Check sheet for the modelled part. Datum: model origin and axes. Units: mm. A direction names the side the tool comes from. Coordinates: 2 decimals unless noted, no trailing zeros. Write each loop counter-clockwise with the first axis right and the second up, starting at its lowest first coordinate (ties: lowest second). Pieces come first, ordered by that corner, then holes. Notation, with made-up numbers: (25.25, 12.5) - (44.25, 12.5) arc R24 ccw to (44.25, 51.5) - close; hole circle Ø9 at (-26.5, -31.75). An arc over 180 degrees is marked (long way). Use one line per item in the form item = value. Start each with the question number.
1. Tool access check on faces 4 (the face through (14, 15.57, 0.99)), 5 (the face through (7.5, 5, 4)), 6 (the face through (-7.5, 5, 4)), 7 (the face through (-9, 21, 10)). Record the directions out of +Z, -Z, +X, -X, +Y, -Y that give a thin tool (end or side, any length) a straight path to the whole face; none if there is none.
2. Cross-section at C-C on x = 0. Record the boundary of the cut face in (y, z).
3. Cross-section at D-D on z = 3.25. Record the boundary of the cut face in (x, y).
4. Cross-section at A-A on z = 16. Record the boundary of the cut face in (x, y).
5. Scan lines: line 1 along Y through (x, z) = (-15.5, 1.55); line 2 along Y through (x, z) = (-3.5, 4.5); line 3 along Y through (x, z) = (-17, 10.5). Record each from-to range of solid material in increasing order.
6. Draft check along Y on faces 1 (the face through (-21, 0, 19)), 2 (the face through (0, 2, 2)), 3 (the face through (0, -23, 10)). Enter one of: +Y half, -Y half, draft (parallel to the pull), parting line (faces both ways), or undercut.
7. Cross-section at B-B on y = 0. Record the boundary of the cut face in (x, z).
8. Go/stop test with flat-tipped pins: pin 1 Ø2.5 at (x, y) = (15.5, 15.5) entering from -Z; pin 2 Ø2 at (y, z) = (5.5, 4) entering from -X; pin 3 Ø1 at (x, z) = (-3, 4) entering from +Y. Record where each tip stops, or that it passes through.
```python
from build123d import *

# Parameters (mm, degrees)
F0_W     = 42
F0_H     = 46
F0_R     = 1.5
F1_DEPTH = 2
F2_W     = 12
F2_H     = 3
F2_W_2   = 42
F3_DEPTH = 16
F4_W     = 42
F4_H     = 46
F4_R     = 2
F4_R_2   = 18
F5_DEPTH = 2
F6_W     = 15
F6_H     = 2
F7_DEPTH = 4
F8_SIZE  = 0.5


with BuildPart() as f1:
    # F0 (on Top) → F1 (new body)
    with BuildSketch(Plane.XY):
        Rectangle(F0_W, F0_H)
        with Locations((-15.5, -15.5)):
            Circle(F0_R, mode=Mode.SUBTRACT)
        with Locations((15.5, -15.5)):
            Circle(F0_R, mode=Mode.SUBTRACT)
        with Locations((-15.5, 15.5)):
            Circle(F0_R, mode=Mode.SUBTRACT)
        with Locations((15.5, 15.5)):
            Circle(F0_R, mode=Mode.SUBTRACT)
    extrude(amount=F1_DEPTH)

    # F2 (on face) → F3 (join)
    with BuildSketch(Plane.XY.offset(2)):
        with Locations((15, 21.5)):
            Rectangle(F2_W, F2_H)
        with Locations((-15, 21.5)):
            Rectangle(F2_W, F2_H)
        with Locations((0, -21.5)):
            Rectangle(F2_W_2, F2_H)
    extrude(amount=F3_DEPTH)

    # F4 (on face) → F5 (join)
    with BuildSketch(Plane.XY.offset(18)):
        Rectangle(F4_W, F4_H)
        with Locations((-16, -18)):
            Circle(F4_R, mode=Mode.SUBTRACT)
        with Locations((16, -18)):
            Circle(F4_R, mode=Mode.SUBTRACT)
        with Locations((-16, 18)):
            Circle(F4_R, mode=Mode.SUBTRACT)
        Circle(F4_R_2, mode=Mode.SUBTRACT)
        with Locations((16, 18)):
            Circle(F4_R, mode=Mode.SUBTRACT)
    extrude(amount=F5_DEPTH)

    # F6 (on face) → F7 (join)
    with BuildSketch(Plane.XY.offset(2)):
        with Locations((0, 9)):
            Rectangle(F6_W, F6_H)
        with Locations((0, 5.5)):
            Rectangle(F6_W, F6_H)
    extrude(amount=F7_DEPTH)

    # F8
    f8_edges = [f1.edges().sort_by_distance(p)[0] for p in [
        (0, 8, 6),
        (0, 6.5, 6),
    ]]
    chamfer(f8_edges, length=F8_SIZE)


solid = f1.part
```
Final values:
q1.face_4 = -Z
q1.face_5 = +Z, +X, +Y
q1.face_6 = +Z, -X, +Y
q1.face_7 = +Y
q2.outline = (-23, 0) - (23, 0) - (23, 2) - (10, 2) - (10, 6) - (8.5, 6) - (8, 5.5) - (8, 2) - (6.5, 2) - (6.5, 5.5) - (6, 6) - (4.5, 6) - (4.5, 2) - (-20, 2) - (-20, 18) - (-18, 18) - (-18, 20) - (-23, 20) - close; (18, 18) - (23, 18) - (23, 20) - (18, 20) - close
q3.outline = (-21, -23) - (21, -23) - (21, -20) - (-21, -20) - close; (-21, 20) - (-9, 20) - (-9, 23) - (-21, 23) - close; (-7.5, 4.5) - (7.5, 4.5) - (7.5, 6.5) - (-7.5, 6.5) - close; (-7.5, 8) - (7.5, 8) - (7.5, 10) - (-7.5, 10) - close; (9, 20) - (21, 20) - (21, 23) - (9, 23) - close
q4.outline = (-21, -23) - (21, -23) - (21, -20) - (-21, -20) - close; (-21, 20) - (-9, 20) - (-9, 23) - (-21, 23) - close; (9, 20) - (21, 20) - (21, 23) - (9, 23) - close
q5.line_1 = -23 to -17, -14 to 14, 17 to 23
q5.line_2 = -23 to -20, 4.5 to 6.5, 8 to 10
q5.line_3 = -23 to -20, 20 to 23
q6.face_1 = draft
q6.face_2 = undercut
q6.face_3 = -Y half
q7.outline = (-21, 0) - (21, 0) - (21, 2) - (-21, 2) - close; (-21, 18) - (-18, 18) - (-18, 20) - (-21, 20) - close; (18, 18) - (21, 18) - (21, 20) - (18, 20) - close
q8.pin_1 = 18
q8.pin_2 = -7.5
q8.pin_3 = 10
